```python
from build123d import *

# Parameters (mm, degrees)
BOSS_EXTRUDE1_DEPTH = 10
BOSS_EXTRUDE2_START = -10
SKETCH3_R           = 2.5
SKETCH3_R_2         = 2
BOSS_EXTRUDE2_DEPTH = 10
MOVE_FACE1_BY       = 5
SKETCH4_R           = 2.5
SKETCH4_R_2         = 1.5
BOSS_EXTRUDE3_DEPTH = 5
SKETCH5_R           = 1.5
CUT_EXTRUDE1_DEPTH  = 5
MOVE_FACE2_BY       = 1
SKETCH11_R          = 1.5
CUT_EXTRUDE2_DEPTH  = 0.75
SKETCH12_R          = 1.5
CUT_EXTRUDE3_DEPTH  = 0.75
FILLET1_R           = 1
SKETCH13_W          = 8
SKETCH13_H          = 3
CUT_EXTRUDE4_DEPTH  = 0.75
SKETCH14_W          = 8
SKETCH14_H          = 3
CUT_EXTRUDE5_DEPTH  = 0.75
BOSS_EXTRUDE6_START = 1
SKETCH16_R          = 2.5
SKETCH16_R_2        = 1.5
BOSS_EXTRUDE6_DEPTH = 1
FILLET3_R           = 2


with BuildPart() as part:
    # Sketch2 → Boss-Extrude1 (new body)
    with BuildSketch(Plane(origin=(0, 0, 0), x_dir=(1, 0, 0), z_dir=(0, 1, 0))):
        with BuildLine():
            Line((0, -1.5), (0, 0))
            Line((0, 0), (-12, 0))
            ThreePointArc((-12, 0), (-12.177124344, -0.822875656), (-12.677124344, -1.5))
            Line((-12.677124344, -1.5), (0, -1.5))
        make_face()
        with BuildLine():
            Line((-12, 0), (0, 0))
            Line((0, 0), (0, 1.5))
            Line((0, 1.5), (-12.677124344, 1.5))
            ThreePointArc((-12.677124344, 1.5), (-12.177124344, 0.822875656), (-12, 0))
        make_face()
        with BuildLine():
            ThreePointArc((-12.677124344, -1.5), (-12.177124344, -0.822875656), (-12, 0))
            Line((-12, 0), (-12.5, 0))
            ThreePointArc((-12.5, 0), (-12.544954729, -0.364476691), (-12.677124344, -0.707106781))
            Line((-12.677124344, -0.707106781), (-12.677124344, -1.5))
        make_face()
        with BuildLine():
            Line((-12.5, 0), (-12, 0))
            ThreePointArc((-12, 0), (-12.177124344, 0.822875656), (-12.677124344, 1.5))
            Line((-12.677124344, 1.5), (-12.677124344, 0.707106781))
            ThreePointArc((-12.677124344, 0.707106781), (-12.544954729, 0.364476691), (-12.5, 0))
        make_face()
        with BuildLine():
            Line((-12.677124344, 0.707106781), (-12.677124344, 1.5))
            ThreePointArc((-12.677124344, 1.5), (-13.292893219, 1.870828693), (-14, 2))
            Line((-14, 2), (-14, 1.5))
            ThreePointArc((-14, 1.5), (-13.228851562, 1.286596318), (-12.677124344, 0.707106781))
        make_face()
        with BuildLine():
            ThreePointArc((-14, -2), (-13.292893219, -1.870828693), (-12.677124344, -1.5))
            Line((-12.677124344, -1.5), (-12.677124344, -0.707106781))
            ThreePointArc((-12.677124344, -0.707106781), (-13.228851562, -1.286596318), (-14, -1.5))
            Line((-14, -1.5), (-14, -2))
        make_face()
        with BuildLine():
            Line((-14, 1.5), (-14, 2))
            ThreePointArc((-14, 2), (-15.414213562, 1.414213562), (-16, 0))
            Line((-16, 0), (-15.5, 0))
            ThreePointArc((-15.5, 0), (-15.060660172, 1.060660172), (-14, 1.5))
        make_face()
        with BuildLine():
            ThreePointArc((-16, 0), (-15.414213562, -1.414213562), (-14, -2))
            Line((-14, -2), (-14, -1.5))
            ThreePointArc((-14, -1.5), (-15.060660172, -1.060660172), (-15.5, 0))
            Line((-15.5, 0), (-16, 0))
        make_face()
    extrude(amount=BOSS_EXTRUDE1_DEPTH)

    # Sketch3 → Boss-Extrude2 (add)
    with BuildSketch(Plane(origin=(0, 10, 0), x_dir=(1, 0, 0), z_dir=(0, 1, 0)).offset(BOSS_EXTRUDE2_START)):
        with Locations((-14, 0)):
            Circle(SKETCH3_R)
        with Locations((-14, 0)):
            Circle(SKETCH3_R_2, mode=Mode.SUBTRACT)
    extrude(amount=BOSS_EXTRUDE2_DEPTH)

    # Move Face1: a face moved inward by 5.0
    extrude(part.faces().sort_by_distance((-7.989839666, 10, 0))[0], amount=MOVE_FACE1_BY, dir=(0, -1, 0), mode=Mode.SUBTRACT)

    # Sketch4 → Boss-Extrude3 (add)
    with BuildSketch(Plane(origin=(0, 5, 0), x_dir=(1, 0, 0), z_dir=(0, 1, 0))):
        Circle(SKETCH4_R)
        Circle(SKETCH4_R_2, mode=Mode.SUBTRACT)
    extrude(amount=-BOSS_EXTRUDE3_DEPTH)

    # Sketch5 → Cut-Extrude1 (cut)
    with BuildSketch(Plane(origin=(0, 5, 0), x_dir=(1, 0, 0), z_dir=(0, 1, 0))):
        with Locations(Location((0, 0, 0), (0, 0, 270))):
            Circle(SKETCH5_R)
    extrude(amount=-CUT_EXTRUDE1_DEPTH, mode=Mode.SUBTRACT)

    # Move Face2: a face moved inward by 1.0
    extrude(part.faces().sort_by_distance((-7, 5, 0))[0], amount=MOVE_FACE2_BY, dir=(0, -1, 0), mode=Mode.SUBTRACT)

    # Sketch11 → Cut-Extrude2 (cut)
    # profile 1 of 2: a face of its own
    with BuildSketch(Plane(origin=(0, 4, 0), x_dir=(1, 0, 0), z_dir=(0, 1, 0))):
        with BuildLine():
            Line((-11, 0), (-11, 1.5))
            Line((-11, 1.5), (-12, 1.5))
            ThreePointArc((-12, 1.5), (-16.5, 0), (-12, -1.5))
            Line((-12, -1.5), (-11, -1.5))
            Line((-11, -1.5), (-11, 0))
        make_face()
        with Locations(Location((-14, 0, 0), (0, 0, 270))):
            Circle(SKETCH11_R, mode=Mode.SUBTRACT)
    # profile 2 of 2: a face of its own
    with BuildSketch(Plane(origin=(0, 4, 0), x_dir=(1, 0, 0), z_dir=(0, 1, 0))):
        with BuildLine():
            Line((-2, 1.5), (-3, 1.5))
            Line((-3, 1.5), (-3, 0))
            Line((-3, 0), (-3, -1.5))
            Line((-3, -1.5), (-2, -1.5))
            ThreePointArc((-2, -1.5), (2.5, 0), (-2, 1.5))
        make_face()
        with Locations(Location((0, 0, 0), (0, 0, 270))):
            Circle(SKETCH11_R, mode=Mode.SUBTRACT)
    extrude(amount=-CUT_EXTRUDE2_DEPTH, mode=Mode.SUBTRACT)

    # Sketch12 → Cut-Extrude3 (cut)
    # profile 1 of 2: a face of its own
    with BuildSketch(Plane(origin=(0, 0, 0), x_dir=(-1, 0, 0), z_dir=(0, -1, 0))):
        with BuildLine():
            Line((11, 1.5), (11, -1.5))
            Line((11, -1.5), (12, -1.5))
            ThreePointArc((12, -1.5), (16.5, 0), (12, 1.5))
            Line((12, 1.5), (11, 1.5))
        make_face()
        with Locations(Location((14, 0, 0), (0, 0, 90))):
            Circle(SKETCH12_R, mode=Mode.SUBTRACT)
    # profile 2 of 2: a face of its own
    with BuildSketch(Plane(origin=(0, 0, 0), x_dir=(-1, 0, 0), z_dir=(0, -1, 0))):
        with BuildLine():
            Line((2, -1.5), (3, -1.5))
            Line((3, -1.5), (3, 1.5))
            Line((3, 1.5), (2, 1.5))
            ThreePointArc((2, 1.5), (-2.5, 0), (2, -1.5))
        make_face()
        with Locations(Location((0, 0, 0), (0, 0, 270))):
            Circle(SKETCH12_R, mode=Mode.SUBTRACT)
    extrude(amount=-CUT_EXTRUDE3_DEPTH, mode=Mode.SUBTRACT)

    # Fillet1
    # the kernel refuses this fillet: 1 mm, written as the material it takes off along each edge
    with BuildSketch(Plane(origin=(-3, 0, 3.920614591), x_dir=(0, 1, 0), z_dir=(0, 0, -1))) as fillet1_piece_1:
        with BuildLine():
            CenterArc((1, -0.968245837), FILLET1_R, 104.477512186, 75.522487814)
            Line((0, -0.968245837), (-0.02, -0.968245837))
            Line((-0.02, -0.968245837), (-0.02, 0))
            Line((-0.02, 0), (0, 0.02))
            ThreePointArc((0, 0.02), (0.375, 0.02), (0.745, 0.019364917))
            Line((0.745, 0.019364917), (0.75, 0))
        make_face()
    extrude(amount=7.841229183, mode=Mode.SUBTRACT)
    with BuildSketch(Plane(origin=(-3, 4, 3.920614591), x_dir=(-1, 0, 0), z_dir=(0, 0, -1))) as fillet1_piece_2:
        with BuildLine():
            CenterArc((0.968245837, -1), FILLET1_R, 90, 75.522487814)
            Line((0, -0.75), (-0.019364917, -0.745))
            ThreePointArc((-0.019364917, -0.745), (-0.02, -0.375), (-0.02, 0))
            Line((-0.02, 0), (0, 0.02))
            Line((0, 0.02), (0.968245837, 0.02))
            Line((0.968245837, 0.02), (0.968245837, 0))
        make_face()
    extrude(amount=7.841229183, mode=Mode.SUBTRACT)
    with BuildSketch(Plane(origin=(-11, 0, -3.920614591), x_dir=(1, 0, 0), z_dir=(0, 0, 1))) as fillet1_piece_3:
        with BuildLine():
            CenterArc((0.968245837, 1), FILLET1_R, 194.477512186, 75.522487814)
            Line((0, 0.75), (-0.019364917, 0.745))
            ThreePointArc((-0.019364917, 0.745), (-0.02, 0.375), (-0.02, 0))
            Line((-0.02, 0), (0, -0.02))
            Line((0, -0.02), (0.968245837, -0.02))
            Line((0.968245837, -0.02), (0.968245837, 0))
        make_face()
    extrude(amount=7.841229183, mode=Mode.SUBTRACT)
    with BuildSketch(Plane(origin=(-11, 4, -3.920614591), x_dir=(0, -1, 0), z_dir=(0, 0, 1))) as fillet1_piece_4:
        with BuildLine():
            CenterArc((1, 0.968245837), FILLET1_R, 180, 75.522487814)
            Line((0, 0.968245837), (-0.02, 0.968245837))
            Line((-0.02, 0.968245837), (-0.02, 0))
            Line((-0.02, 0), (0, -0.02))
            ThreePointArc((0, -0.02), (0.375, -0.02), (0.745, -0.019364917))
            Line((0.745, -0.019364917), (0.75, 0))
        make_face()
    extrude(amount=7.841229183, mode=Mode.SUBTRACT)

    # Sketch13 → Cut-Extrude4 (cut)
    with BuildSketch(Plane(origin=(0, 0, 0), x_dir=(-1, 0, 0), z_dir=(0, -1, 0))):
        with Locations((7, 0)):
            Rectangle(SKETCH13_W, SKETCH13_H)
    extrude(amount=-CUT_EXTRUDE4_DEPTH, mode=Mode.SUBTRACT)

    # Sketch14 → Cut-Extrude5 (cut)
    with BuildSketch(Plane(origin=(0, 4, 0), x_dir=(1, 0, 0), z_dir=(0, 1, 0))):
        with Locations((-7, 0)):
            Rectangle(SKETCH14_W, SKETCH14_H)
    extrude(amount=-CUT_EXTRUDE5_DEPTH, mode=Mode.SUBTRACT)

    # Sketch16 → Boss-Extrude6 (add)
    with BuildSketch(Plane(origin=(0, 0.75, 0), x_dir=(-1, 0, 0), z_dir=(0, -1, 0)).offset(BOSS_EXTRUDE6_START)):
        with Locations(Location((14, 0, 0), (0, 0, 216.869897646))):
            Circle(SKETCH16_R)
        with Locations(Location((14, 0, 0), (0, 0, 90))):
            Circle(SKETCH16_R_2, mode=Mode.SUBTRACT)
    extrude(amount=-BOSS_EXTRUDE6_DEPTH)

    # Fillet3
    # the kernel refuses this fillet: 2 mm, written as the material it adds along each edge
    with BuildSketch(Plane(origin=(-14, 0.75, 0), x_dir=(-0.720984929131136, 0, -0.6929507428134924), z_dir=(-0.6929507428134924, 0, 0.720984929131136))) as fillet3_piece_1_section:
        with BuildLine():
            CenterArc((4.232050808, 2), FILLET3_R, 210, 60)
            Line((4.232050808, 0), (4.232050808, -0.04))
            Line((4.232050808, -0.04), (2.5, -0.04))
            Line((2.5, -0.04), (2.46, 0))
            ThreePointArc((2.46, 0), (2.46, 0.5), (2.465358984, 0.98))
            Line((2.465358984, 0.98), (2.5, 1))
        make_face()
    fillet3_piece_1 = revolve(axis=Axis((-14, 0.75, 0), (0, -1, 0)), revolution_arc=272.27171598, mode=Mode.PRIVATE)
    fillet3_piece_1 = split(fillet3_piece_1, bisect_by=Plane(origin=(-11.214858776, 0.489042262, 1.5), z_dir=(0, 0, -1)), keep=Keep.TOP, mode=Mode.PRIVATE)
    fillet3_piece_1 = split(fillet3_piece_1, bisect_by=Plane(origin=(-11.214858776, 0.489042262, -1.5), z_dir=(0, 0, 1)), keep=Keep.TOP, mode=Mode.PRIVATE)
    add(fillet3_piece_1)


solid = part.part
```
The listing builds one solid part. Answer for the finished solid, in the listing's coordinates (mm). A direction names the side the tool comes from. Give positions to 0.01 mm unless a question says otherwise; leave off trailing zeros. Order: outer loops, then holes, each group sorted by start corner. A loop starts at its lowest first (then second) coordinate and runs counter-clockwise, first axis right, second up. Notation, with made-up numbers: (36.25, 42.25) - (67.25, 42.25) arc R30 ccw to (67.25, 71.25) - close; hole circle Ø4 at (84, 22.25). An arc over 180 degrees is marked (long way). Answer in a Markdown table with one row per item. Add a question column.
Q1. The part is cut by section B-B (y = 0.2). Determine the outline of the cut face in (x, z).
Q2. Find the intervals of material crossed by line 1 along X through (y, z) = (0.85, 0); line 2 along Z through (x, y) = (0, 1.6); line 3 along X through (y, z) = (2.5, 0.95), in increasing order. Write a range as [from, to].
Q3. For a pull along X with two mould halves and no side action, classify faces 3 (the flat face through (-7, 2, -1.5)), 4 (the flat face through (-4, 0.75, 0)) as released by +X, released by -X, zero draft, split by the parting line, or undercut.
Q4. The part is cut by section C-C (x = -4.75). Determine the outline of the cut face in (y, z), then the cut area to 3 significant figures.
Q5. The part is cut by section A-A (y = 2). Determine the outline of the cut face in (x, z).
Q6. Which of the six approach directions +Z, -Z, +X, -X, +Y, -Y give full straight-line access (tool end or side, diameter ignored) to faces 1 (the flat face through (-12, -0.25, 0)), 2 (the flat face through (-7, 2, 1.5))?
Q7. Given P1, Ø1.5, axis at x = -13, y = 2.5, coming from the +Z side; P2, Ø2.5, axis at x = -3.5, z = 0, coming from the -Y side; P3, Ø2.5, axis at x = -14, z = 0, coming from the -Y side; P4, Ø1, axis at y = 1.5, z = -1, coming from the -X side, each flat-ended and moving along its own axis, determine where each tip first touches the part or whether it passes through.
Determined:
| question | item | result |
|---|---|---|
| 1 | outline | (-12, -1.5) - (-11.57, -1.5) arc R2.85 ccw to (-11.57, 1.5) - (-12, 1.5) arc R2.5 ccw (long way) to start; hole circle Ø3 at (-14, 0) |
| 2 | line 1 | x = [-16.5, -15.5], [-12.5, -1.5], [1.5, 2.5] |
| 2 | line 2 | z = [-2.5, -1.5], [1.5, 2.5] |
| 2 | line 3 | x = [-16.31, -15.16], [-12.84, -1.16], [1.16, 2.31] |
| 3 | face 3 | undercut |
| 3 | face 4 | zero draft |
| 4 | outline | (0.75, -1.5) - (3.25, -1.5) - (3.25, 1.5) - (0.75, 1.5) - close |
| 4 | area | 7.50 mm² |
| 5 | outline | (-12, -1.5) - (-2, -1.5) arc R2.5 ccw (long way) to (-2, 1.5) - (-12, 1.5) arc R2.5 ccw (long way) to start; hole circle Ø3 at (-14, 0); hole circle Ø3 at (0, 0) |
| 6 | face 1 | +Z, -Z, +X, -X, -Y |
| 6 | face 2 | +Z, +Y, -Y |
| 7 | P1 | stops at z = 2.49 |
| 7 | P2 | stops at y = 0.75 |
| 7 | P3 | passes through |
| 7 | P4 | stops at x = -16.45 |
